```python
from build123d import *

# Parameters (mm, degrees)
EXTRUDE_1_DEPTH          = 4
SKETCH_3_W               = 4
SKETCH_3_H               = 1.8
EXTRUDE_2_DEPTH          = 5.5
SKETCH_5_W               = 4
SKETCH_5_H               = 3
EXTRUDE_3_DEPTH          = 3.7
MIRROR_3_COPY_1_SKETCH_W = 4
MIRROR_3_COPY_1_SKETCH_H = 3
MIRROR_3_COPY_1_DEPTH    = 3.7
SKETCH_7_W               = 4
SKETCH_7_H               = 2
EXTRUDE_4_DEPTH          = 3
MIRROR_5_COPY_1_SKETCH_W = 4
MIRROR_5_COPY_1_SKETCH_H = 2
MIRROR_5_COPY_1_DEPTH    = 3


with BuildPart() as part:
    # Эскиз2 → Бобышка-Вытянуть1 (new, symmetric)
    with BuildSketch(Plane.XY):
        with BuildLine():
            Line((0, 0), (0, 0.9))
            Line((0, 0.9), (4, 0.9))
            ThreePointArc((4, 0.9), (5.226251594, 0.551100379), (6.5, 0.605771366))
            Line((6.5, 0.605771366), (11, 8.4))
            Line((11, 8.4), (13.5, 8.4))
            Line((13.5, 8.4), (13.5, -8.4))
            Line((13.5, -8.4), (11, -8.4))
            Line((11, -8.4), (6.5, -0.605771366))
            ThreePointArc((6.5, -0.605771366), (5.226251594, -0.551100379), (4, -0.9))
            Line((4, -0.9), (0, -0.9))
            Line((0, -0.9), (0, 0))
        make_face()
    extrude(amount=EXTRUDE_1_DEPTH, both=True)

    # Эскиз3 → Бобышка-Вытянуть2 (add)
    with BuildSketch(Plane(origin=(0, 0, -4), x_dir=(-1, 0, 0), z_dir=(0, 0, -1))):
        with Locations((-2, 0)):
            Rectangle(SKETCH_3_W, SKETCH_3_H)
    extrude_2 = extrude(amount=EXTRUDE_2_DEPTH)

    # Зеркальное отражение1: Бобышка-Вытянуть2 across plane
    add(extrude_2.mirror(Plane.XY))

    # Эскиз5 → Бобышка-Вытянуть3 (add)
    with BuildSketch(Plane(origin=(0, 0.9, 0), x_dir=(1, 0, 0), z_dir=(0, 1, 0))):
        with Locations((2, 8)):
            Rectangle(SKETCH_5_W, SKETCH_5_H)
    extrude_3 = extrude(amount=EXTRUDE_3_DEPTH)

    # Зеркальное отражение2: Бобышка-Вытянуть3 across plane
    add(extrude_3.mirror(Plane.XY))

    # Зеркальное отражение3: Бобышка-Вытянуть3 across plane
    add(extrude_3.mirror(Plane.ZX))

    # Зеркальное отражение3 copy 1 sketch → Зеркальное отражение3 copy 1 (add)
    with BuildSketch(Plane.XZ.offset(0.9)):
        with Locations((2, 8)):
            Rectangle(MIRROR_3_COPY_1_SKETCH_W, MIRROR_3_COPY_1_SKETCH_H)
    extrude(amount=MIRROR_3_COPY_1_DEPTH)

    # Эскиз7 → Бобышка-Вытянуть4 (add)
    with BuildSketch(Plane(origin=(0, 0, 6.5), x_dir=(-1, 0, 0), z_dir=(0, 0, -1))):
        with Locations((-2, 3.6)):
            Rectangle(SKETCH_7_W, SKETCH_7_H)
    extrude_4 = extrude(amount=EXTRUDE_4_DEPTH)

    # Зеркальное отражение4: Бобышка-Вытянуть4 across plane
    add(extrude_4.mirror(Plane.XY))

    # Зеркальное отражение5: Бобышка-Вытянуть4 across plane
    add(extrude_4.mirror(Plane.ZX))

    # Зеркальное отражение5 copy 1 sketch → Зеркальное отражение5 copy 1 (add)
    with BuildSketch(Plane(origin=(0, 0, -6.5), x_dir=(-1, 0, 0), z_dir=(0, 0, 1))):
        with Locations((-2, 3.6)):
            Rectangle(MIRROR_5_COPY_1_SKETCH_W, MIRROR_5_COPY_1_SKETCH_H)
    extrude(amount=MIRROR_5_COPY_1_DEPTH)


solid = part.part
```
Model file for the job. Use its own axes, mm. A direction names the side the tool comes from. Coordinates: 2 decimals unless noted, no trailing zeros. Loops run counter-clockwise (first coordinate to the right, second up) from the corner with the lowest first, then second, coordinate; pieces in that order, holes last. Notation, with made-up numbers: M 13.5,85 L 46.5,85 A23 cw 46.5,107 Z; hole C 71.5,79 d10. An arc over 180 degrees is marked long. Use CSV: the item, a comma, the result in double quotes. Start each with the question number.
1. Tool access for faces 5 (the flat face through (2, -2, -6.5)), 6 (the flat face through (2, 0, -9.5)), 7 (the flat face through (2, -4, -3.5)), 8 (the flat face through (11, 0, 4)): list every direction of +Z, -Z, +X, -X, +Y, -Y with a clear straight run to the whole face (end or side of a thin tool).
2. Flat gauge pins, fed straight in: pin 1 (3.5 mm diameter, centred on x = 2, z = 5, fed in from -Y); pin 2 (5 mm diameter, centred on x = 9, z = 0.5, fed in from -Y); pin 3 (1 mm diameter, centred on x = 8, y = -2, fed in from +Z); pin 4 (3 mm diameter, centred on x = 1, z = 7.5, fed in from +Y). Where does each tip first touch, or does it go through?
3. Two-plate mould, pull along Y, no slides. Class faces 1 (the flat face through (13.5, 0, 0)), 2 (the flat face through (2, 0.9, 0)), 3 (the flat face through (2, 2, 6.5)), 4 (the flat face through (8.72, 4.45, 0.06)): pulls with the +Y half, pulls with the -Y half, needs draft (parallel to the pull), parting line crosses it, or undercut.
4. Band-saw the part on A-A, the plane z = 4.75. List the corners of the cut face in (x, y), then the cut area to 3 significant figures.
5. Band-saw the part on B-B, the plane y = 3.25. List the corners of the cut face in (x, z).
6. Band-saw the part on D-D, the plane z = -2. List the corners of the cut face in (x, y), then the cut area to 3 significant figures.
7. Probe probe 1 along Y at (x, z) = (1, -5); probe 2 along Z at (x, y) = (0.5, -2.5); probe 3 along Z at (x, y) = (3, 3.5). List the from-to ranges inside material, lowest first. Write a range as [from, to].
8. Band-saw the part on C-C, the plane x = 3.5. List the corners of the cut face in (y, z).
Entries:
1,face 5,"+X, -X"
1,face 6,"-Z, +X, -X, +Y, -Y"
1,face 7,"-X, -Y"
1,face 8,"+Z, +X, +Y, -Y"
2,pin 1,"stops at y = -4.6"
2,pin 2,"stops at y = -8.4"
2,pin 3,"stops at z = 4"
2,pin 4,"stops at y = 4.6"
3,face 1,"needs draft"
3,face 2,"undercut"
3,face 3,"undercut"
3,face 4,"pulls with the +Y half"
4,outline,"M 0,-4.6 L 4,-4.6 L 4,-2.6 L 0,-2.6 Z; M 0,-0.9 L 4,-0.9 L 4,0.9 L 0,0.9 Z; M 0,2.6 L 4,2.6 L 4,4.6 L 0,4.6 Z"
4,area,"23.2 mm2"
5,outline,"M 0,-9.5 L 4,-9.5 L 4,-3.5 L 0,-3.5 Z; M 0,3.5 L 4,3.5 L 4,9.5 L 0,9.5 Z; M 8.03,-4 L 13.5,-4 L 13.5,4 L 8.03,4 Z"
6,outline,"M 0,-0.9 L 4,-0.9 A4 cw 6.5,-0.61 L 11,-8.4 L 13.5,-8.4 L 13.5,8.4 L 11,8.4 L 6.5,0.61 A4 cw 4,0.9 L 0,0.9 Z"
6,area,"92.8 mm2"
7,probe 1,"y = [-4.6, -2.6], [-0.9, 0.9], [2.6, 4.6]"
7,probe 2,"z = [-9.5, -6.5], [6.5, 9.5]"
7,probe 3,"z = [-9.5, -3.5], [3.5, 9.5]"
8,outline,"M -4.6,-9.5 L 4.6,-9.5 L 4.6,-3.5 L 2.6,-3.5 L 2.6,-6.5 L 0.9,-6.5 L 0.9,6.5 L 2.6,6.5 L 2.6,3.5 L 4.6,3.5 L 4.6,9.5 L -4.6,9.5 L -4.6,3.5 L -2.6,3.5 L -2.6,6.5 L -0.9,6.5 L -0.9,-6.5 L -2.6,-6.5 L -2.6,-3.5 L -4.6,-3.5 Z"
